The drawing under review shows one solid part. Ordinate dimensions are in mm from its lowest x, y, z. A direction names the side the tool comes from. Give positions to 0.01 mm unless a question says otherwise; leave off trailing zeros. Order: outer loops, then holes, each group sorted by start corner. A loop starts at its lowest first (then second) coordinate and runs counter-clockwise, first axis right, second up. Notation, with made-up numbers: (-29, -13.75) -> (11, -13.75) arc R17 cw to (11, 5.25) -> close; hole circle Ø11 at (10, -34.75). An arc over 180 degrees is marked (long way). One line per item, written item: value.
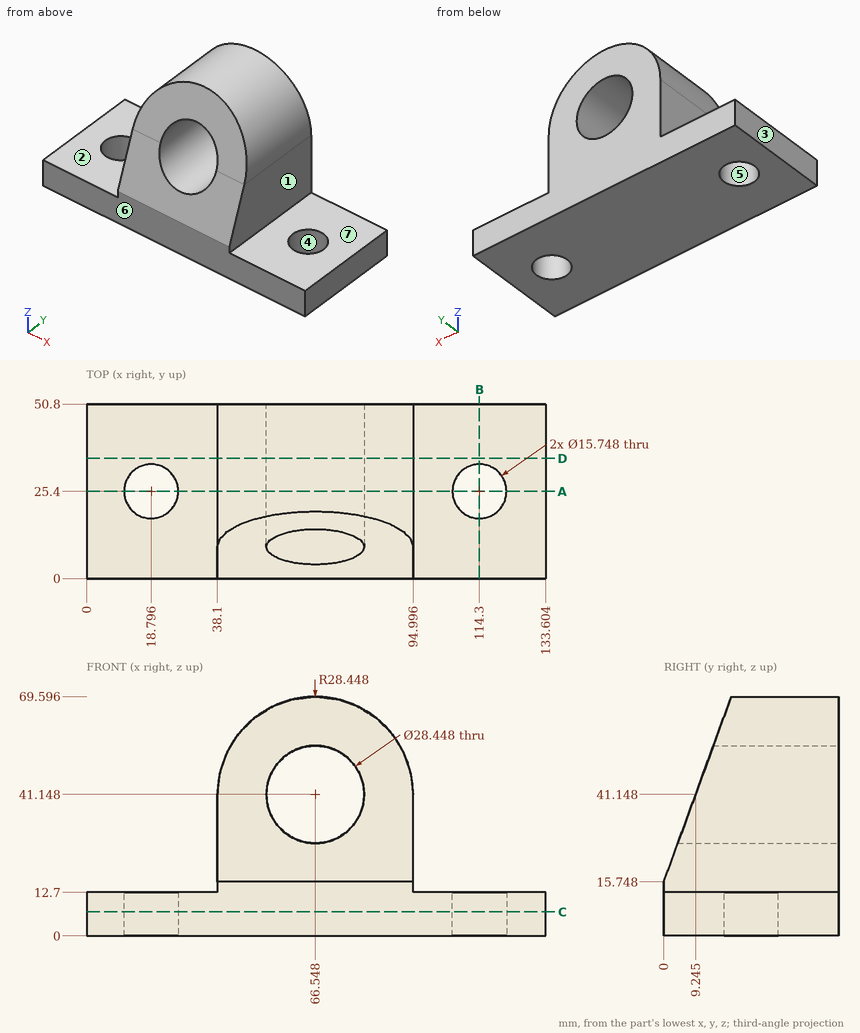
Item 1: Add section A-A on y = 25.4. Give the boundary of the cut face in (x, z), plus the area to 3 significant figures.
Returned:
outline: (0, 0) -> (10.92, 0) -> (10.92, 12.7) -> (0, 12.7) -> close; (26.67, 0) -> (106.43, 0) -> (106.43, 12.7) -> (95, 12.7) -> (95, 41.15) arc R28.45 ccw to (38.1, 41.15) -> (38.1, 12.7) -> (26.67, 12.7) -> close; (122.17, 0) -> (133.6, 0) -> (133.6, 12.7) -> (122.17, 12.7) -> close; hole circle Ø28.45 at (66.55, 41.15)
area: 3,550 mm²
Item 2: To check wall thickness, follow line 1 along Y through (x, z) = (114, 10); line 2 along X through (y, z) = (38, 32); line 3 along X through (y, z) = (12.5, 15). State the ranges of each line that lie inside material, in increasing order. Write a range as from..to.
Returned:
line 1: 0..17.53, 33.27..50.8
line 2: 38.1..55.66, 77.44..95
line 3: 38.1..95
Item 3: Add section C-C on z = 7. Give the boundary of the cut face in (x, y).
Returned:
outline: (0, 0) -> (133.6, 0) -> (133.6, 50.8) -> (0, 50.8) -> close; hole circle Ø15.75 at (18.8, 25.4); hole circle Ø15.75 at (114.3, 25.4)
Item 4: Add section B-B on x = 114.3. Give the boundary of the cut face in (y, z).
Returned:
outline: (0, 0) -> (17.53, 0) -> (17.53, 12.7) -> (0, 12.7) -> close; (33.27, 0) -> (50.8, 0) -> (50.8, 12.7) -> (33.27, 12.7) -> close
Item 5: Machinability: for the marked faces 1, 2 and 3, which of the approach directions +Z, -Z, +X, -X, +Y, -Y give a long, thin tool a straight path to every point of the face, cutting with its end or side? Answer none if there is none.
Returned:
face 1: +Z, +X, +Y, -Y
face 2: +Z, -X, +Y, -Y
face 3: +Z, -Z, -X, +Y, -Y
Item 6: Add section D-D on y = 35. Give the boundary of the cut face in (x, z), plus the area to 3 significant figures.
Returned:
outline: (0, 0) -> (133.6, 0) -> (133.6, 12.7) -> (95, 12.7) -> (95, 41.15) arc R28.45 ccw to (38.1, 41.15) -> (38.1, 12.7) -> (0, 12.7) -> close; hole circle Ø28.45 at (66.55, 41.15)
area: 3,950 mm²
Item 7: Clearance check with flat-ended pins moving along their axes: P1, Ø8, axis at x = 91.5, z = 20.5, coming from the -Y side; P2, Ø8, axis at y = 6.5, z = 24, coming from the -X side; P3, Ø2, axis at x = 75.5, z = 62, coming from the -Y side; P4, Ø14, axis at x = 18.796, y = 25.4, coming from the +Z side. State where each tip first meets the part, or that it passes through.
Returned:
P1: y = 0.27
P2: x = 38.1
P3: y = 16.47
P4: through
Item 8: Draft analysis for pull direction Y (two halves, no side actions). For the marked faces 4, 5, 6 and 7, state which applies: pulls with the +Y half, pulls with the -Y half, needs draft (parallel to the pull), parting line crosses it, or undercut.
Returned:
face 4: undercut
face 5: undercut
face 6: pulls with the -Y half
face 7: needs draft
